Here's the drawing with two shaded views (mm, measured from the low corner). I have some questions. Coordinates: 2 decimals unless noted, no trailing zeros. Write each loop counter-clockwise with the first axis right and the second up, starting at its lowest first coordinate (ties: lowest second). Pieces come first, ordered by that corner, then holes. Notation, with made-up numbers: (8, 24) - (22, 24) arc R9 cw to (22, 32) - close; hole circle Ø8 at (37, 59.5). An arc over 180 degrees is marked (long way). Answer in a Markdown table with one row per item. Add a question column.
Item 1: If I drill on probe 1 along X at (y, z) = (2.95, 40); probe 2 along Z at (x, y) = (46.5, 0.7) (1 decimal); probe 3 along X at (y, z) = (1, 19), over which ranges is the centre line in solid material (lowest first)? Write a range as from..to.
Item 2: Imagine slicing it at C-C (y = 1.3). State how many separate pieces and enclosed holes the cut face has, plus the area to 3 significant figures.
Item 3: Imagine slicing it at B-B (z = 38). Please give me the cut outline in (x, y) (1 decimal).
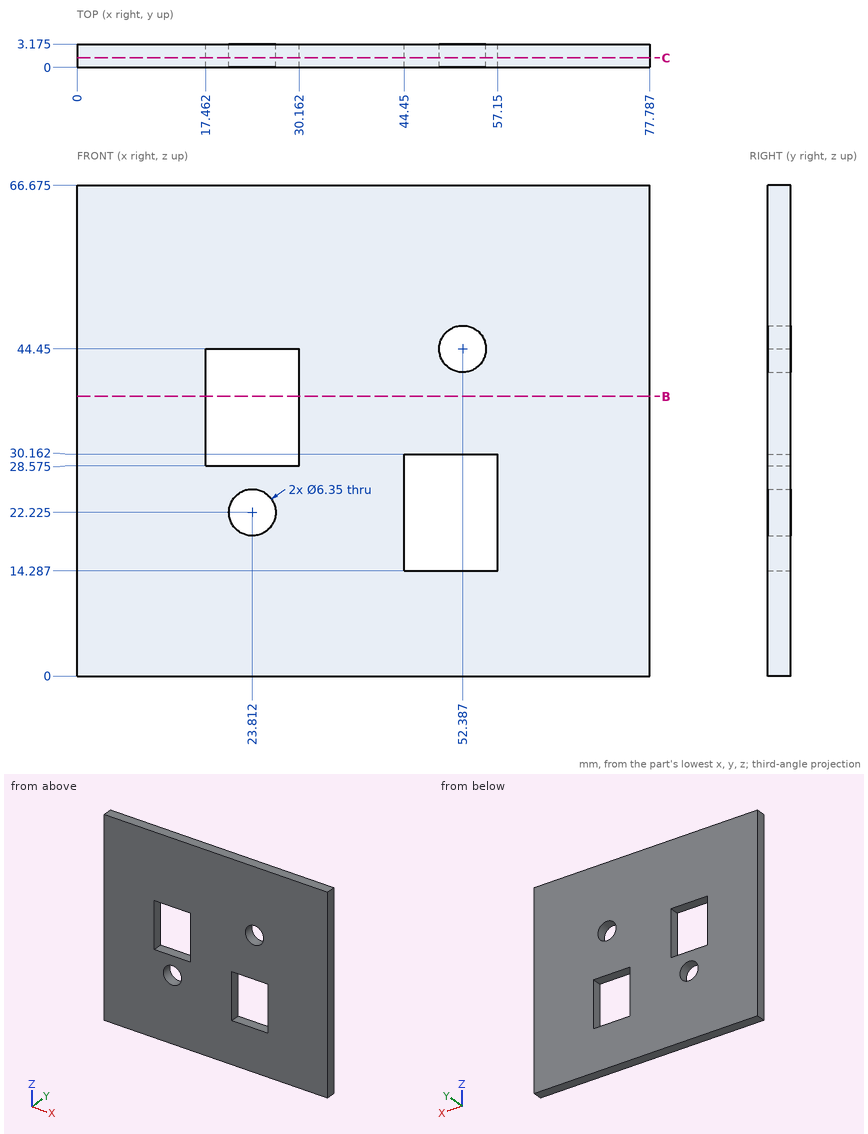
Here are the results:
| question | item | result |
|---|---|---|
| 1 | probe 1 | x = 0..17.46, 30.16..77.79 |
| 1 | probe 2 | z = 0..14.3, 30.2..66.7 |
| 1 | probe 3 | x = 0..44.45, 57.15..77.79 |
| 2 | separate pieces | 1 |
| 2 | enclosed holes | 4 |
| 2 | area | 4,720 mm2 |
| 3 | outline | (0, 0) - (17.5, 0) - (17.5, 3.2) - (0, 3.2) - close; (30.2, 0) - (77.8, 0) - (77.8, 3.2) - (30.2, 3.2) - close |
